Source: CAD feature listing. Evaluate the final solid. Frame: model axes, mm. Round coordinates to 2 decimals unless told otherwise and drop trailing zeros. Loops run counter-clockwise (first coordinate to the right, second up) from the corner with the lowest first, then second, coordinate; pieces in that order, holes last. Notation, with made-up numbers: (82, 34.25) - (96, 34.25) arc R14 ccw to (96, 40.25) - close; hole circle Ø5 at (-13.5, 63.25). An arc over 180 degrees is marked (long way). Use CSV: the item, a comma, the result in double quotes. Start each with the question number.
from build123d import *

# Parameters (mm, degrees)
F0_W     = 80
F0_H     = 260
F0_R     = 2
F0_R_2   = 4.25
F1_DEPTH = 12


with BuildPart() as f1:
    # F0 (on Top) → F1 (new body)
    with BuildSketch(Plane.XY):
        Rectangle(F0_W, F0_H)
        with Locations((-36, -115)):
            Circle(F0_R, mode=Mode.SUBTRACT)
        with Locations((-36, -89)):
            Circle(F0_R, mode=Mode.SUBTRACT)
        with Locations((-10, -115)):
            Circle(F0_R, mode=Mode.SUBTRACT)
        with Locations((-10, -89)):
            Circle(F0_R, mode=Mode.SUBTRACT)
        with Locations((-20, 60)):
            Circle(F0_R_2, mode=Mode.SUBTRACT)
        with Locations((-36, 89)):
            Circle(F0_R, mode=Mode.SUBTRACT)
        with Locations((-36, 115)):
            Circle(F0_R, mode=Mode.SUBTRACT)
        with Locations((-10, 89)):
            Circle(F0_R, mode=Mode.SUBTRACT)
        with Locations((-10, 115)):
            Circle(F0_R, mode=Mode.SUBTRACT)
        with Locations((20, 60)):
            Circle(F0_R_2, mode=Mode.SUBTRACT)
    extrude(amount=F1_DEPTH)


solid = f1.part
1. Mould query, pull axis Y, two halves, no side actions, for faces 1 (the flat face through (-1, 130, 6)), 2 (the cylindrical face through (-20.92, 55.85, 5.92)), 3 (the flat face through (-1, 2, 12)). Classes: +Y half, -Y half, draft (parallel to the pull), parting line (faces both ways), or undercut.
2. Line query: line 1 along Y through (x, z) = (-10, 5.75); line 2 along Y through (x, z) = (18, 2.5); line 3 along Y through (x, z) = (17, 4). Output: solid intervals per line, ascending.
3. Section query A-A on x = 20. Return the cut outline in (y, z), and give its area (3 significant figures).
Values:
1,face 1,"+Y half"
1,face 2,"undercut"
1,face 3,"draft"
2,line 1,"y = -130 to -117, -113 to -91, -87 to 87, 91 to 113, 117 to 130"
2,line 2,"y = -130 to 56.25, 63.75 to 130"
2,line 3,"y = -130 to 56.99, 63.01 to 130"
3,outline,"(-130, 0) - (55.75, 0) - (55.75, 12) - (-130, 12) - close; (64.25, 0) - (130, 0) - (130, 12) - (64.25, 12) - close"
3,area,"3,020 mm^2"
